Verification items for this drawing (mm, ordinates from the low corner). Round coordinates to 2 decimals unless told otherwise and drop trailing zeros. Write each loop counter-clockwise with the first axis right and the second up, starting at its lowest first coordinate (ties: lowest second). Pieces come first, ordered by that corner, then holes.
Item 1: Depth check by flat-ended pin: P1, Ø2, axis at y = 64, z = 1.5, coming from the -X side; P2, Ø1.1, axis at y = 175.5, z = 3.5, coming from the -X side; P3, Ø2.5, axis at y = 185, z = 3.95, coming from the +X side. Enter the tip coordinate at first touch or a pass-through.
Item 2: Scan lines: probe 1 along Y at (x, z) = (4, 3.95); probe 2 along Z at (x, y) = (3.85, 185); probe 3 along Y at (x, z) = (7, 4). Record each from-to range of solid material in increasing order.
Item 3: Cross-section at A-A (y = 166.5). Enter the section's corners in (x, z).
Item 4: Cross-section at C-C (y = 16.5). Enter the section's corners in (x, z), then the cut area to 3 significant figures.
Item 5: Cross-section at B-B (x = 1.5). Enter the section's corners in (y, z).
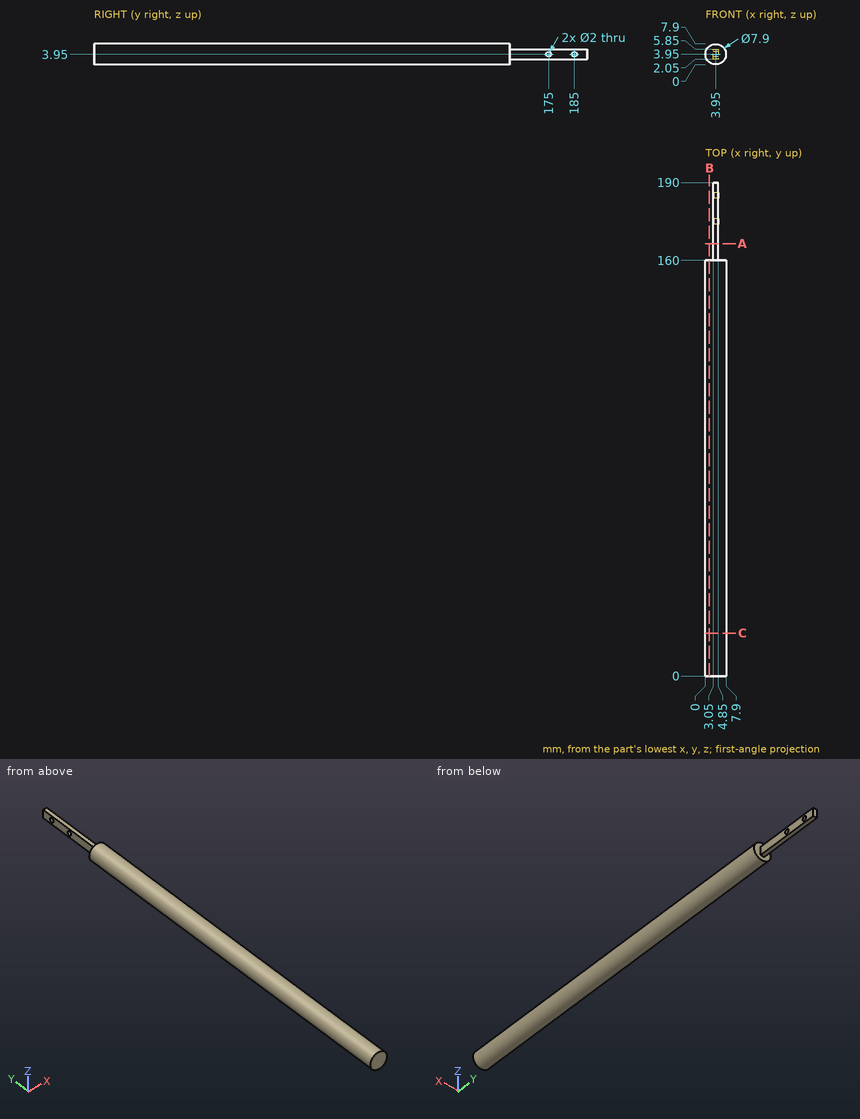
Resolved:
1. P1: stops at x = 0.28
1. P2: stops at x = 3.05
1. P3: stops at x = 4.85
2. probe 1: y = 0 to 174, 176 to 184, 186 to 190
2. probe 2: z = 2.05 to 2.95, 4.95 to 5.85
2. probe 3: y = 0 to 160
3. outline: (3.05, 2.05) - (4.85, 2.05) - (4.85, 5.85) - (3.05, 5.85) - close
4. outline: circle Ø7.9 at (3.95, 3.95)
4. area: 49.0 mm2
5. outline: (0, 0.85) - (160, 0.85) - (160, 7.05) - (0, 7.05) - close
